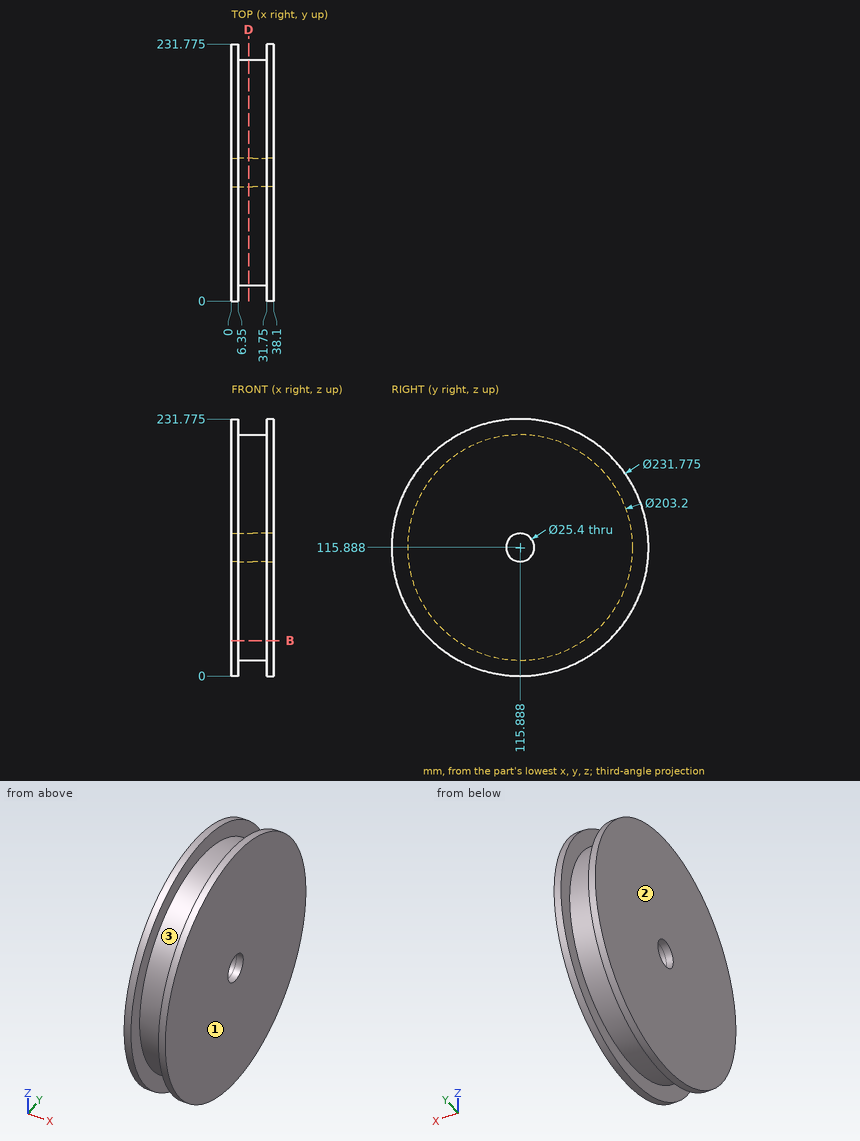
The drawing under review shows one solid part. Ordinate dimensions are in mm from its lowest x, y, z. Coordinates: 2 decimals unless noted, no trailing zeros. Order: outer loops, then holes, each group sorted by start corner. A loop starts at its lowest first (then second) coordinate and runs counter-clockwise, first axis right, second up. Notation, with made-up numbers: (27.25, 4.5) - (33.25, 4.5) arc R10 cw to (33.25, 15.5) - close; hole circle Ø5 at (0.25, -31.5). An arc over 180 degrees is marked (long way). Put each result on its own line as item: value.
1) The part is to be moulded in two halves that separate along X. For the marked faces 1, 2 and 3, say which applies: released by +X, released by -X, zero draft, split by the parting line, or undercut.
Response values:
face 1: released by +X
face 2: released by -X
face 3: undercut
2) Take a section at D-D, the plane x = 15.5. Give the boundary of the cut face in (y, z).
Response values:
outline: circle Ø203.2 at (115.89, 115.89); hole circle Ø25.4 at (115.89, 115.89)
3) Insertion check: P1, Ø2, axis at x = 4.5, z = 144.5, coming from the +Y side; P2, Ø2, axis at x = 11, z = 57.5, coming from the -Y side; P3, Ø12, axis at x = 17.5, z = 76, coming from the +Y side. Each pin has a flat end and moves straight along its axis. Give the tip position at first contact, or say it passes through.
Response values:
P1: stops at y = 228.44
P2: stops at y = 32.05
P3: stops at y = 211.67
4) Wall thickness on L1, parallel to X at y = 163.5, z = 25; L2, parallel to Z at x = 33.5, y = 117 (1 decimal); L3, parallel to Y at x = 9, z = 107 (1 decimal): over which ranges is each line inside the solid? List them lowest first. Write a range as from..to.
Response values:
L1: x = 0..6.35, 31.75..38.1
L2: z = 0..103.2, 128.5..231.8
L3: y = 14.7..106.8, 125..217.1
5) Take a section at B-B, the plane z = 32. Give the boundary of the cut face in (x, y), and give its area (3 significant figures).
Response values:
outline: (0, 35.93) - (6.35, 35.93) - (6.35, 58.57) - (31.75, 58.57) - (31.75, 35.93) - (38.1, 35.93) - (38.1, 195.84) - (31.75, 195.84) - (31.75, 173.21) - (6.35, 173.21) - (6.35, 195.84) - (0, 195.84) - close
area: 4,940 mm²
